Input: dimensioned drawing with shaded views. Units: mm. Origin: part minimum x, y, z. Give positions to 0.01 mm unless a question says otherwise; leave off trailing zeros. Order: outer loops, then holes, each group sorted by start corner. A loop starts at its lowest first (then second) coordinate and runs counter-clockwise, first axis right, second up.
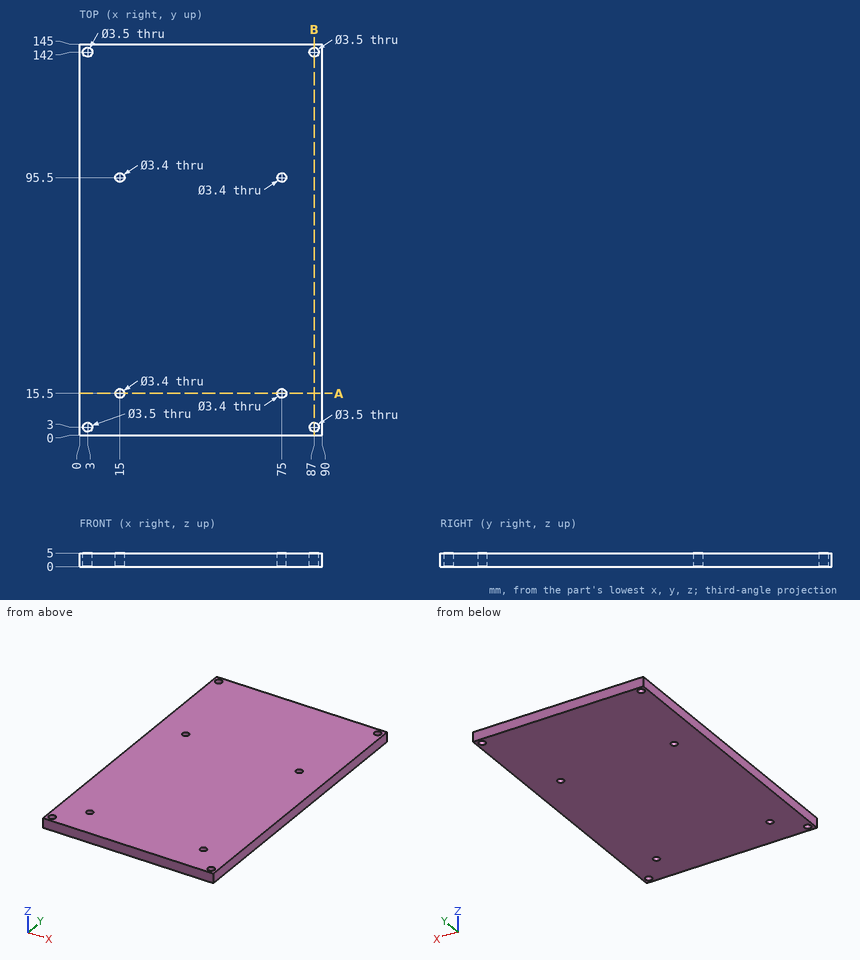
1) Section query A-A, the plane y = 15.5. Return the cut outline in (x, z), and give its area (3 significant figures).
Report:
outline: (0, 0) - (13.3, 0) - (13.3, 5) - (0, 5) - close; (16.7, 0) - (73.3, 0) - (73.3, 5) - (16.7, 5) - close; (76.7, 0) - (90, 0) - (90, 5) - (76.7, 5) - close
area: 416 mm2
2) Material intervals for L1, parallel to Y at x = 3, z = 1.4; L2, parallel to Y at x = 15, z = 2; L3, parallel to X at y = 95.5, z = 1.6, sorted ascending.
Report:
L1: y = 0 to 1.25, 4.75 to 140.25, 143.75 to 145
L2: y = 0 to 13.8, 17.2 to 93.8, 97.2 to 145
L3: x = 0 to 13.3, 16.7 to 73.3, 76.7 to 90
3) Section query B-B, the plane x = 87. Return the cut outline in (y, z), and give its area (3 significant figures).
Report:
outline: (0, 0) - (1.25, 0) - (1.25, 5) - (0, 5) - close; (4.75, 0) - (140.25, 0) - (140.25, 5) - (4.75, 5) - close; (143.75, 0) - (145, 0) - (145, 5) - (143.75, 5) - close
area: 690 mm2
